Here's how the part is built. I have some questions about the finished solid (model axes, mm). Face numbers are marked on the shaded views. A direction names the side the tool comes from. Round coordinates to 2 decimals unless told otherwise and drop trailing zeros. Loops run counter-clockwise (first coordinate to the right, second up) from the corner with the lowest first, then second, coordinate; pieces in that order, holes last. Notation, with made-up numbers: (-18, -31.75) - (12, -31.75) arc R10 cw to (12, -12.75) - close; hole circle Ø1 at (12, 53.5). An arc over 180 degrees is marked (long way). Answer as a JSON object with one key per item and string values. Group by question number.
1) I want a section at A-A, the plane z = -92. Please give me the cut outline in (x, y), then the cut area to 3 significant figures.
2) I want a section at D-D, the plane x = 18. Please give me the cut outline in (y, z), then the cut area to 3 significant figures.
3) I want a section at B-B, the plane y = 8. Please give me the cut outline in (x, z), then the cut area to 3 significant figures.
4) Will these pins go through, and if not, where does the flat tip stop? P1, Ø12, axis at y = -9.5, z = -2, coming from the +X side; P2, Ø17.5, axis at x = -2, z = 11.5, coming from the -Y side; P3, Ø8, axis at y = 24, z = -5.5, coming from the +X side; P4, Ø18, axis at x = -0.5, y = -5.5, coming from the -Z side.
5) If we mould it in two halves opening along X, with no side actions, what happens to the marked faces 1, 2 and 3? For each: pulls with the +X half, pulls with the -X half, needs draft (parallel to the pull), parting line crosses it, or undercut.
6) Which directions (+Z, -Z, +X, -X, +Y, -Y) give clear straight access to the entire face, cutting with the end or side of a thin tool? Please do the marked faces 4 and 5.
7) If I drill on line 1 along X through (y, z) = (-16.65, 16.84); line 2 along X through (y, z) = (-6, -21); line 3 along X through (y, z) = (-16, 16), over which ranges is the centre line in solid material (lowest first)? Write a range as [from, to].
8) I want a section at C-C, the plane y = -5. Please give me the cut outline in (x, z).
from build123d import *

# Parameters (mm, degrees)
BOSS_EXTRUDE1_DEPTH = 22
M16_TAPPED_HOLE1_D  = 14
BOSS_EXTRUDE2_DEPTH = 96
CUT_EXTRUDE1_DEPTH  = 127.957167334
SKETCH8_W           = 64
SKETCH8_H           = 52
BOSS_EXTRUDE3_DEPTH = 26
CHAMFER1_SIZE       = 16
SKETCH11_R          = 3
BOSS_EXTRUDE4_DEPTH = 4


with BuildPart() as part:
    # Sketch1 → Boss-Extrude1 (new body)
    with BuildSketch(Plane.XY):
        with BuildLine():
            Line((-31.551158378, -1.471617029), (-31.551158378, -18.121617029))
            Line((-31.551158378, -18.121617029), (32.448841622, -18.121617029))
            Line((32.448841622, -18.121617029), (32.448841622, -1.471617029))
            Line((32.448841622, -1.471617029), (30.752510469, -1.471617029))
            ThreePointArc((30.752510469, -1.471617029), (29.21725341, -1.04901606), (28.114530432, 0.099725795))
            Line((28.114530432, 0.099725795), (15.257528673, 23.839860621))
            Line((15.257528673, 23.839860621), (13.614601967, 26.873484031))
            ThreePointArc((13.614601967, 26.873484031), (0.448841622, 33.78157804), (-12.716918722, 26.873484031))
            Line((-12.716918722, 26.873484031), (-14.359845428, 23.839860621))
            Line((-14.359845428, 23.839860621), (-27.216847187, 0.099725795))
            ThreePointArc((-27.216847187, 0.099725795), (-28.319570165, -1.04901606), (-29.854827224, -1.471617029))
            Line((-29.854827224, -1.471617029), (-31.551158378, -1.471617029))
        make_face()
    extrude(amount=BOSS_EXTRUDE1_DEPTH)

    # M16 Tapped Hole1 (through all)
    with Locations(Plane.XY.offset(22)):
        with Locations((0.448841622, 17.78157804)):
            Hole(M16_TAPPED_HOLE1_D / 2)

    # Sketch4 → Boss-Extrude2 (add)
    with BuildSketch(Plane.XY):
        Polygon((16.448841622, -18.121617029), (16.448841622, -10.121617029), (8.448841622, -10.121617029), (8.448841622, -1.471617029), (32.448841622, -1.471617029), (32.448841622, -18.121617029), align=None)
        Polygon((-7.551158378, -10.121617029), (-7.551158378, -1.471617029), (-31.551158378, -1.471617029), (-31.551158378, -18.121617029), (-15.551158378, -18.121617029), (-15.551158378, -10.121617029), align=None)
    extrude(amount=-BOSS_EXTRUDE2_DEPTH)

    # Sketch5 → Cut-Extrude1 (cut, through all)
    with BuildSketch(Plane.XY.offset(22)):
        Polygon((-15.551158378, -18.121617029), (16.448841622, -18.121617029), (16.448841622, -10.121617029), (8.448841622, -10.121617029), (8.448841622, -1.471617029), (-7.551158378, -1.471617029), (-7.551158378, -10.121617029), (-15.551158378, -10.121617029), align=None)
    extrude(amount=-CUT_EXTRUDE1_DEPTH, mode=Mode.SUBTRACT)

    # Sketch8 → Boss-Extrude3 (add)
    with BuildSketch(Plane(origin=(0, 0, -96), x_dir=(-1, 0, 0), z_dir=(0, 0, -1))):
        with Locations((-0.448841622, 7.878382971)):
            Rectangle(SKETCH8_W, SKETCH8_H)
    extrude(amount=BOSS_EXTRUDE3_DEPTH)

    # Chamfer1
    chamfer1_edges = [part.edges().sort_by_distance(p)[0] for p in [
        (0.448841622, 33.878382971, -122),
    ]]
    chamfer(chamfer1_edges, length=CHAMFER1_SIZE)

    # Sketch11 → Boss-Extrude4 (add)
    # profile 1 of 4: a face of its own
    with BuildSketch(Plane(origin=(0, -18.121617029, 0), x_dir=(-1, 0, 0), z_dir=(0, -1, 0))):
        with BuildLine():
            Line((-32.448841622, -22), (-39.588841622, -22))
            ThreePointArc((-39.588841622, -22), (-42.417268747, -20.828427125), (-43.588841622, -18))
            Line((-43.588841622, -18), (-43.588841622, -15.68))
            ThreePointArc((-43.588841622, -15.68), (-42.417268747, -12.851572875), (-39.588841622, -11.68))
            Line((-39.588841622, -11.68), (-32.448841622, -11.68))
            Line((-32.448841622, -11.68), (-32.448841622, -22))
        make_face()
        with Locations(Location((-38.018841622, -16.84, 0), (0, 0, 90))):
            Circle(SKETCH11_R, mode=Mode.SUBTRACT)
    # profile 2 of 4: a face of its own
    with BuildSketch(Plane(origin=(0, -18.121617029, 0), x_dir=(-1, 0, 0), z_dir=(0, -1, 0))):
        with BuildLine():
            Line((31.551158378, -11.68), (38.691158378, -11.68))
            ThreePointArc((38.691158378, -11.68), (41.519585502, -12.851572875), (42.691158378, -15.68))
            Line((42.691158378, -15.68), (42.691158378, -18))
            ThreePointArc((42.691158378, -18), (41.519585502, -20.828427125), (38.691158378, -22))
            Line((38.691158378, -22), (31.551158378, -22))
            Line((31.551158378, -22), (31.551158378, -11.68))
        make_face()
        with Locations(Location((37.121158378, -16.84, 0), (0, 0, 270))):
            Circle(SKETCH11_R, mode=Mode.SUBTRACT)
    # profile 3 of 4: a face of its own
    with BuildSketch(Plane(origin=(0, -18.121617029, 0), x_dir=(-1, 0, 0), z_dir=(0, -1, 0))):
        with BuildLine():
            Line((-32.448841622, 112.43498208), (-39.588841622, 112.43498208))
            ThreePointArc((-39.588841622, 112.43498208), (-42.417268747, 113.606554955), (-43.588841622, 116.43498208))
            Line((-43.588841622, 116.43498208), (-43.588841622, 118.75498208))
            ThreePointArc((-43.588841622, 118.75498208), (-42.417268747, 121.583409205), (-39.588841622, 122.75498208))
            Line((-39.588841622, 122.75498208), (-32.448841622, 122.75498208))
            Line((-32.448841622, 122.75498208), (-32.448841622, 112.43498208))
        make_face()
        with Locations(Location((-38.018841622, 117.59498208, 0), (0, 0, 270))):
            Circle(SKETCH11_R, mode=Mode.SUBTRACT)
    # profile 4 of 4: a face of its own
    with BuildSketch(Plane(origin=(0, -18.121617029, 0), x_dir=(-1, 0, 0), z_dir=(0, -1, 0))):
        with BuildLine():
            Line((31.551158378, 122.75498208), (31.551158378, 112.43498208))
            Line((31.551158378, 112.43498208), (38.691158378, 112.43498208))
            ThreePointArc((38.691158378, 112.43498208), (41.519585502, 113.606554955), (42.691158378, 116.43498208))
            Line((42.691158378, 116.43498208), (42.691158378, 118.75498208))
            ThreePointArc((42.691158378, 118.75498208), (41.519585502, 121.583409205), (38.691158378, 122.75498208))
            Line((38.691158378, 122.75498208), (31.551158378, 122.75498208))
        make_face()
        with Locations(Location((37.121158378, 117.59498208, 0), (0, 0, 90))):
            Circle(SKETCH11_R, mode=Mode.SUBTRACT)
    extrude(amount=-BOSS_EXTRUDE4_DEPTH)


solid = part.part
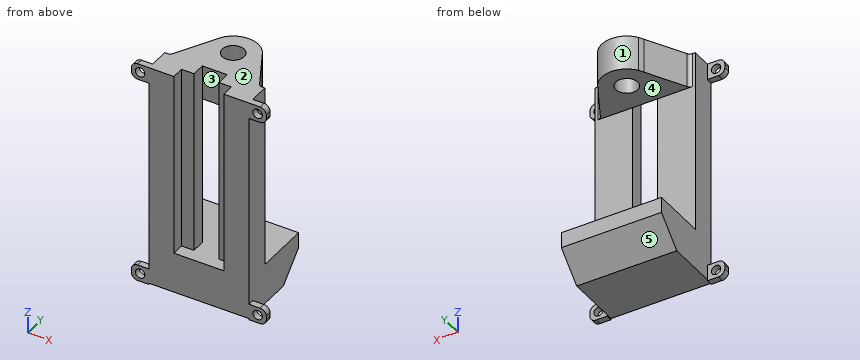
Outcome:
{
 "1": {"outline": "(-31.55, -18.12) - (-15.55, -18.12) - (-15.55, -10.12) - (-7.55, -10.12) - (-7.55, -1.47) - (-31.55, -1.47) - close; (8.45, -10.12) - (16.45, -10.12) - (16.45, -18.12) - (32.45, -18.12) - (32.45, -1.47) - (8.45, -1.47) - close", "area": "671 mm^2"},
 "2": {"outline": "(-18.12, -122) - (17.88, -122) - (33.88, -106) - (33.88, -96) - (-1.47, -96) - (-1.47, 0) - (18.78, 0) - (18.78, 22) - (-18.12, 22) - close", "area": "3,630 mm^2"},
 "3": {"outline": "(-31.55, -122) - (32.45, -122) - (32.45, -96) - (-31.55, -96) - close; (-22.94, 0) - (23.84, 0) - (23.84, 22) - (-22.94, 22) - close", "area": "2,690 mm^2"},
 "4": {"P1": "x = 32.45", "P2": "y = -10.12", "P3": "through", "P4": "z = -122"},
 "5": {"face 1": "parting line crosses it", "face 2": "needs draft", "face 3": "undercut"},
 "6": {"face 4": "+X, -X, +Y", "face 5": "-Z, +X, -X, +Y"},
 "7": {"line 1": "[-42.69, -40.12], [-34.12, -15.55], [16.45, 35.02], [41.02, 43.59]", "line 2": "[-31.55, -7.55], [8.45, 32.45]", "line 3": "[-42.69, -40], [-34.24, -15.55], [16.45, 35.14], [40.9, 43.59]"},
 "8": {"outline": "(-31.55, -122) - (32.45, -122) - (32.45, 22) - (8.45, 22) - (8.45, -96) - (-7.55, -96) - (-7.55, 22) - (-31.55, 22) - close"}
}
